Check sheet for the modelled part. Datum: model origin and axes. Units: mm. Face numbers are marked on the shaded views. A direction names the side the tool comes from. Round coordinates to 2 decimals unless told otherwise and drop trailing zeros. Write each loop counter-clockwise with the first axis right and the second up, starting at its lowest first coordinate (ties: lowest second). Pieces come first, ordered by that corner, then holes. Notation, with made-up numbers: (17, 58.5) -> (21, 58.5) arc R21 ccw to (21, 88.5) -> close; hole circle Ø7 at (-34.5, -22.75). An arc over 180 degrees is marked (long way). One line per item, written item: value.
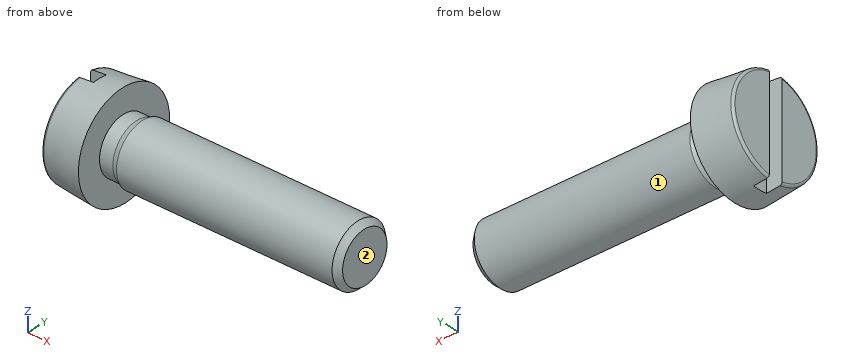
Autodesk Inventor part; units mm, degrees
ref_plane "Work Plane1" through (30.1625, 0, 0) normal (0, 0, -1) x (1, 0, 0)
ref_plane "YZ Plane" through (0, 0, 0) normal (1, 0, 0) x (0, 1, 0)
ref_plane "XZ Plane" through (0, 0, 0) normal (0, 1, 0) x (-1, 0, 0)
sketch "Sketch1" plane through (0, 0, 0) normal (0, 0, 1) x (1, 0, 0)
  line L0 (-3.3, 0) -> (20, 0)
  line L1 (20, 0) -> (20, 2.5)
  line L2 (20, 2.5) -> (1.6, 2.5)
  line L3 (1.6, 2.5) -> (1.1091, 2.2835)
  line L4 (1.1091, 2.2835) -> (0, 2.2835)
  line L5 (0, 2.2835) -> (0, 4.25)
  line L6 (-7.96, 0) -> (24.66, 0)
  line L7 (0, -0.85) -> (0, 5.1)
  line L8 (-3.3, 0) -> (-3.3, 3.9613)
  line L9 (0, 4.25) -> (-3.3, 3.9613)
  line L10 (1.6, 2.5) -> (0, 2.5) construction
  dimension "d0" = 20
  dimension "d1" = 18.4
  dimension "d2" = 0.4909
  dimension "d3" = 3.3
  dimension "d4" = 5
  dimension "d5" = 4.567
  dimension "d9" = 8.5
  dimension "d10" = 5
revolve "Body" add sketch "Sketch1" angle 360 about axis through (-3.3, 0, 0) along (1, 0, 0)
sketch "Sketch2" plane through (-3.3, 0, 0) normal (-1, 0, 0) x (0, 0, 1)
  circle A0 centre (0, 0) radius 4.25
  line L0 (0, 0) -> (0, 3.9613)
  line L1 (-4.25, 0.6) -> (4.25, 0.6)
  line L2 (4.25, 0.6) -> (4.25, -0.6)
  line L3 (4.25, -0.6) -> (-4.25, -0.6)
  line L4 (-4.25, -0.6) -> (-4.25, 0.6)
  line L5 (-4.25, 0) -> (4.25, 0) construction
  line L6 (0, 0.6) -> (0, -0.6) construction
  point P0 (0, 0)
  dimension "d11" = 1.2
  dimension "d12" = 8.5
fillet "Fillet1" radius 0.2 1 edges at (-3.3, -3.9613, 0)
extrude "Slot" cut sketch "Sketch2" against normal blind 1.3 contours A0 L3 L1 | L2 L3 A0 | A0 L1 L2 | A0 L4 L1 | L3 L4 A0
thread "Thread"
chamfer "Chamfer1" distance 0.433 distance2 0.4909 1 edges at (20, -2.5, 0) measured on face at (20, 1.2612, -0.6619)
ref_plane "Work Plane1" through (30.1625, 0, 0) normal (0, 0, -1) x (1, 0, 0)
equation "\"d11\" = SBR"
equation "\"d12\" = KOD"
equation "\"d14\" = RR"
equation "\"d19\" = STI"
equation "\"d15\" = GEL"
equation "\"d17\" = -0.5 * SPD + 0.5 * GD"
equation "\"d0\" = NLG"
equation "\"d1\" = GEL"
equation "\"d3\" = KOH"
equation "\"d4\" = GD"
equation "\"d5\" = BDM"
equation "\"d9\" = KOD"
equation "\"d10\" = KEWI"
equation "\"GD\" = 5"
equation "\"NLG\" = 20"
equation "\"GEL\" = 18.4"
equation "\"KOD\" = 8.5"
equation "\"KOH\" = 3.3"
equation "\"GAL\" = 0.61345 * PTC"
equation "\"SPD\" = 4.13397"
equation "\"BDM\" = 4.56699"
equation "\"GUL\" = 0.61345 * PTC"
equation "\"RR\" = 0.2"
equation "\"SBR\" = 1.2"
equation "\"STI\" = 1.3"
equation "\"KEWI\" = 5deg"
equation "\"PTC\" = 0.8"
equation "\"THREADDIA\" = 5"
equation "\"TOA\" = 30deg"
equation "\"NND\" = 5"
equation "\"GD1\" = THREADDIA - 1.2269 * PTC"
properties part number "DIN 84 - M5 x 20" material "Steel, Mild"
Item 1: Tool access check on the marked faces 1 and 2. Record the directions out of +Z, -Z, +X, -X, +Y, -Y that give a thin tool (end or side, any length) a straight path to the whole face; none if there is none.
Answer:
face 1: +X
face 2: +Z, -Z, +X, +Y, -Y
Item 2: Sectioned sample at A-A on y = 0. Enter the section's corners in (x, z).
Answer:
outline: (-2, -4.08) -> (0, -4.25) -> (0, -2.28) -> (1.11, -2.28) -> (1.6, -2.5) -> (19.51, -2.5) -> (20, -2.07) -> (20, 2.07) -> (19.51, 2.5) -> (1.6, 2.5) -> (1.11, 2.28) -> (0, 2.28) -> (0, 4.25) -> (-2, 4.08) -> close
Item 3: Sectioned sample at C-C on x = 4.5. Enter the section's corners in (y, z), and give its area (3 significant figures).
Answer:
outline: circle Ø5 at (0, 0)
area: 19.6 mm^2
Item 4: Sectioned sample at B-B on z = 0. Enter the section's corners in (x, y), and give its area (3 significant figures).
Answer:
outline: (-3.3, -3.78) arc R0.2 ccw to (-3.12, -3.98) -> (0, -4.25) -> (0, -2.28) -> (1.11, -2.28) -> (1.6, -2.5) -> (19.51, -2.5) -> (20, -2.07) -> (20, 2.07) -> (19.51, 2.5) -> (1.6, 2.5) -> (1.11, 2.28) -> (0, 2.28) -> (0, 4.25) -> (-3.12, 3.98) arc R0.2 ccw to (-3.3, 3.78) -> (-3.3, 0.6) -> (-2, 0.6) -> (-2, -0.6) -> (-3.3, -0.6) -> close
area: 125 mm^2
Item 5: Depth check by flat-ended pin: P1, Ø0.6, axis at y = 0, z = -0.5, coming from the -X side; P2, Ø5, axis at y = -3, z = 1, coming from the +X side; P3, Ø1.5, axis at x = 12, z = 1, coming from the -Y side; P4, Ø0.7, axis at x = -2.5, z = -0.5, coming from the -Y side. Enter the tip coordinate at first touch or a pass-through.
Answer:
P1: stops at x = -2
P2: stops at x = 20
P3: stops at y = -2.49
P4: stops at y = -4.05
Item 6: Thickness scan on line 1 (X direction, y = -3, z = -1.25); line 2 (X direction, y = -0.25, z = -0.5); line 3 (Z direction, x = 7.25, y = 1.75). Record the ranges inside material, lowest first.
Answer:
line 1: x = -3.3 to 0
line 2: x = -2 to 20
line 3: z = -1.79 to 1.79
